from build123d import *

# Parameters (mm, degrees)
SKETCH1_R           = 22.475
SKETCH1_R_2         = 20
BOSS_EXTRUDE1_DEPTH = 15
SKETCH2_R           = 23.455
SKETCH2_R_2         = 20
BOSS_EXTRUDE2_DEPTH = 1.5
CUT_EXTRUDE3_DEPTH  = 10
CIRPATTERN1_COUNT   = 3
FILLET1_R           = 1


with BuildPart() as part:
    # Sketch1 → Boss-Extrude1 (new body)
    with BuildSketch(Plane(origin=(0, 0, 0), x_dir=(1, 0, 0), z_dir=(0, 1, 0))):
        with Locations(Location((0, 0, 0), (0, 0, 270))):
            Circle(SKETCH1_R)
        with Locations(Location((0, 0, 0), (0, 0, 270))):
            Circle(SKETCH1_R_2, mode=Mode.SUBTRACT)
    extrude(amount=BOSS_EXTRUDE1_DEPTH)

    # Sketch2 → Boss-Extrude2 (add)
    with BuildSketch(Plane.XZ):
        with Locations(Location((0, 0, 0), (0, 0, 270))):
            Circle(SKETCH2_R)
        with Locations(Location((0, 0, 0), (0, 0, 270))):
            Circle(SKETCH2_R_2, mode=Mode.SUBTRACT)
    extrude(amount=BOSS_EXTRUDE2_DEPTH)

    # Sketch4 → Cut-Extrude3 (cut)
    with BuildSketch(Plane(origin=(0, 0, 0), x_dir=(1, 0, 0), z_dir=(0, 1, 0))):
        with BuildLine():
            Line((-11.2375, 19.463921), (-11.7275, 20.312626))
            ThreePointArc((-11.7275, 20.312626), (0, 23.455), (11.7275, 20.312626))
            Line((11.7275, 20.312626), (11.2375, 19.463921))
            ThreePointArc((11.2375, 19.463921), (0, 22.475), (-11.2375, 19.463921))
        make_face()
    cut_extrude3 = extrude(amount=-CUT_EXTRUDE3_DEPTH, mode=Mode.SUBTRACT)

    # CirPattern1: Cut-Extrude3 ×3 about axis
    cirpattern1_axis = Axis((0, 0, 0), (0, 1, 0))
    for i in range(1, CIRPATTERN1_COUNT):
        add(cut_extrude3.rotate(cirpattern1_axis, i * 360 / CIRPATTERN1_COUNT), mode=Mode.SUBTRACT)

    # Fillet1
    fillet1_edges = [part.edges().sort_by_distance(p)[0] for p in [
        (11.2375, -0.75, -19.463921),
        (-11.2375, -0.75, -19.463921),
        (-22.475, -0.75, 0),
        (-11.2375, -0.75, 19.463921),
        (11.2375, -0.75, 19.463921),
        (22.475, -0.75, 0),
    ]]
    fillet(fillet1_edges, radius=FILLET1_R)


solid = part.part
Check sheet for the modelled part. Datum: model origin and axes. Units: mm. A direction names the side the tool comes from. Round coordinates to 2 decimals unless told otherwise and drop trailing zeros. Order: outer loops, then holes, each group sorted by start corner. A loop starts at its lowest first (then second) coordinate and runs counter-clockwise, first axis right, second up.
(1) Go/stop test with flat-tipped pins: P1, Ø1, axis at y = 10.5, z = -15, coming from the -X side; P2, Ø5, axis at y = 7, z = -16, coming from the +X side; P3, Ø8, axis at y = 6.5, z = 15.5, coming from the +X side. Record where each tip stops, or that it passes through.
(2) Scan lines: probe 1 along Z at (x, y) = (0, -0.9) (3 decimals); probe 2 along Z at (x, y) = (0, 9.75) (3 decimals). Record each from-to range of solid material in increasing order.
(3) Cross-section at B-B, the plane z = -7.5. Enter the section's corners in (x, y).
(4) Access from +Z, -Z, +X, -X, +Y, -Y to the whole of each face (thin tool, end or side, straight path). Record for faces 5 (the flat face through (20, 0, -11)), 6 (the cylindrical face through (-20.398, -0.74, -11.578)), 7 (the flat face through (0, 0, 23)).
(5) Cross-section at D-D, the plane x = -15. Enter the section's corners in (y, z).
(6) Cross-section at C-C, the plane y = 12. Enter the section's corners in (x, z) (3 decimals).
(7) Cross-section at A-A, the plane x = 0. Enter the section's corners in (y, z) (3 decimals), and give its area (3 significant figures).
(8) Draft check along Z on faces 1 (the cylindrical face through (-11.13, -0.76, -19.85)), 2 (the cylindrical face through (11.624, -0.76, 19.563)), 3 (the cylindrical face through (-11.624, -0.76, 19.563)), 4 (the flat face through (-1.6, 15, -20.1)). Enter one of: pulls with the +Z half, pulls with the -Z half, needs draft (parallel to the pull), parting line crosses it, or undercut.
Check sheet entries:
1. P1: stops at x = -17.17
1. P2: stops at x = 17.97
1. P3: stops at x = 19.31
2. probe 1: z = -22.475 to -20, 20 to 23.455
2. probe 2: z = -22.475 to -20, 20 to 22.475
3. outline: (-22.22, -1.5) - (-18.54, -1.5) - (-18.54, 15) - (-21.19, 15) - (-21.19, 0) - (-22.22, 0) - close; (18.54, -1.5) - (22.22, -1.5) - (22.22, 0) - (21.19, 0) - (21.19, 15) - (18.54, 15) - close
4. face 5: -Z, +X, +Y
4. face 6: -Z, -X, +Y, -Y
4. face 7: +Z, +Y
5. outline: (-1.5, -18.03) - (0, -18.03) - (0, -16.74) - (15, -16.74) - (15, -13.23) - (-1.5, -13.23) - close; (-1.5, 13.23) - (15, 13.23) - (15, 16.74) - (-1.5, 16.74) - close
6. outline: circle Ø44.95 at (0, 0); hole circle Ø40 at (0, 0)
7. outline: (-1.5, -22.475) - (15, -22.475) - (15, -20) - (-1.5, -20) - close; (-1.5, 20) - (15, 20) - (15, 22.475) - (0, 22.475) - (0, 23.455) - (-1.5, 23.455) - close
7. area: 83.1 mm2
8. face 1: pulls with the -Z half
8. face 2: undercut
8. face 3: undercut
8. face 4: needs draft
